from build123d import *

# Parameters (mm, degrees)
SKETCH_1_W          = 120
SKETCH_1_H          = 45
SKETCH_1_R          = 2.6
EXTRUDE_1_DEPTH     = 20
FILLET_1_R          = 10
CUT_EXTRUDE_1_DEPTH = 10


with BuildPart() as part:
    # 草图1 → 凸台-拉伸1 (new body)
    with BuildSketch(Plane.XY):
        Rectangle(SKETCH_1_W, SKETCH_1_H)
        with Locations((-50.8, 12.7)):
            Circle(SKETCH_1_R, mode=Mode.SUBTRACT)
        with Locations((-50.8, 0)):
            Circle(SKETCH_1_R, mode=Mode.SUBTRACT)
        with Locations((-50.8, -12.7)):
            Circle(SKETCH_1_R, mode=Mode.SUBTRACT)
        with Locations((-38.1, 12.7)):
            Circle(SKETCH_1_R, mode=Mode.SUBTRACT)
        with Locations((-38.1, 0)):
            Circle(SKETCH_1_R, mode=Mode.SUBTRACT)
        with Locations((-38.1, -12.7)):
            Circle(SKETCH_1_R, mode=Mode.SUBTRACT)
        with Locations((-25.4, 12.7)):
            Circle(SKETCH_1_R, mode=Mode.SUBTRACT)
        with Locations((-25.4, 0)):
            Circle(SKETCH_1_R, mode=Mode.SUBTRACT)
        with Locations((-25.4, -12.7)):
            Circle(SKETCH_1_R, mode=Mode.SUBTRACT)
        with Locations((-12.7, 12.7)):
            Circle(SKETCH_1_R, mode=Mode.SUBTRACT)
        with Locations((-12.7, 0)):
            Circle(SKETCH_1_R, mode=Mode.SUBTRACT)
        with Locations((-12.7, -12.7)):
            Circle(SKETCH_1_R, mode=Mode.SUBTRACT)
        with Locations((0, 12.7)):
            Circle(SKETCH_1_R, mode=Mode.SUBTRACT)
        Circle(SKETCH_1_R, mode=Mode.SUBTRACT)
        with Locations((0, -12.7)):
            Circle(SKETCH_1_R, mode=Mode.SUBTRACT)
        with Locations((12.7, 12.7)):
            Circle(SKETCH_1_R, mode=Mode.SUBTRACT)
        with Locations((12.7, 0)):
            Circle(SKETCH_1_R, mode=Mode.SUBTRACT)
        with Locations((12.7, -12.7)):
            Circle(SKETCH_1_R, mode=Mode.SUBTRACT)
        with Locations((25.4, 12.7)):
            Circle(SKETCH_1_R, mode=Mode.SUBTRACT)
        with Locations((25.4, 0)):
            Circle(SKETCH_1_R, mode=Mode.SUBTRACT)
        with Locations((25.4, -12.7)):
            Circle(SKETCH_1_R, mode=Mode.SUBTRACT)
        with Locations((38.1, 12.7)):
            Circle(SKETCH_1_R, mode=Mode.SUBTRACT)
        with Locations((38.1, 0)):
            Circle(SKETCH_1_R, mode=Mode.SUBTRACT)
        with Locations((38.1, -12.7)):
            Circle(SKETCH_1_R, mode=Mode.SUBTRACT)
        with Locations((50.8, 12.7)):
            Circle(SKETCH_1_R, mode=Mode.SUBTRACT)
        with Locations((50.8, 0)):
            Circle(SKETCH_1_R, mode=Mode.SUBTRACT)
        with Locations((50.8, -12.7)):
            Circle(SKETCH_1_R, mode=Mode.SUBTRACT)
    extrude(amount=EXTRUDE_1_DEPTH)

    # 圆角1
    fillet_1_edges = [part.edges().sort_by_distance(p)[0] for p in [
        (60, -22.5, 10),
        (-60, -22.5, 10),
        (-60, 22.5, 10),
        (60, 22.5, 10),
    ]]
    fillet(fillet_1_edges, radius=FILLET_1_R)

    # 草图2 → 切除-拉伸1 (cut)
    with BuildSketch(Plane.XY.offset(20)):
        with BuildLine():
            Line((-60, 5.2), (65.881182767, 5.2))
            ThreePointArc((65.881182767, 5.2), (71.081182767, 0), (65.881182767, -5.2))
            Line((65.881182767, -5.2), (-60, -5.2))
            ThreePointArc((-60, -5.2), (-65.2, 0), (-60, 5.2))
        make_face()
    extrude(amount=-CUT_EXTRUDE_1_DEPTH, mode=Mode.SUBTRACT)


solid = part.part
The model under review builds one solid part; all positions refer to its coordinate system, in mm. A direction names the side the tool comes from. Coordinates: 2 decimals unless noted, no trailing zeros. Write each loop counter-clockwise with the first axis right and the second up, starting at its lowest first coordinate (ties: lowest second). Pieces come first, ordered by that corner, then holes. Notation, with made-up numbers: M 44,21.25 L 73,21.25 A15 ccw 73,40.25 Z; hole C 55.25,62.25 d10. An arc over 180 degrees is marked long. Put each result on its own line as item: value.
1) Add section C-C on x = -31. Give the boundary of the cut face in (y, z), then the cut area to 3 significant figures.
Computed:
outline: M -22.5,0 L 22.5,0 L 22.5,20 L 5.2,20 L 5.2,10 L -5.2,10 L -5.2,20 L -22.5,20 Z
area: 796 mm2
2) Add section B-B on x = -12.7. Give the boundary of the cut face in (y, z).
Computed:
outline: M -22.5,0 L -15.3,0 L -15.3,20 L -22.5,20 Z; M -10.1,0 L -2.6,0 L -2.6,10 L -5.2,10 L -5.2,20 L -10.1,20 Z; M 2.6,0 L 10.1,0 L 10.1,20 L 5.2,20 L 5.2,10 L 2.6,10 Z; M 15.3,0 L 22.5,0 L 22.5,20 L 15.3,20 Z
3) Draft analysis for pull direction Y (two halves, no side actions). For faces 1 (the cylindrical face through (-35.62, -11.92, 9.86)), 2 (the flat face through (-1, -22.5, 10)), 3 (the cylindrical face through (-48.32, 0.78, 4.93)), 4 (the flat face through (-1, 22.5, 10)), state which applies: released by +Y, released by -Y, zero draft, split by the parting line, or undercut.
Computed:
face 1: undercut
face 2: released by -Y
face 3: undercut
face 4: released by +Y
4) Wall thickness on probe 1 along Y at (x, z) = (0, 14); probe 2 along Y at (x, z) = (-38.1, 9.25); probe 3 along Y at (x, z) = (-6.5, 16.25): over which ranges is each line inside the solid? List them lowest first. Write a range as [from, to].
Computed:
probe 1: y = [-22.5, -15.3], [-10.1, -5.2], [5.2, 10.1], [15.3, 22.5]
probe 2: y = [-22.5, -15.3], [-10.1, -2.6], [2.6, 10.1], [15.3, 22.5]
probe 3: y = [-22.5, -5.2], [5.2, 22.5]
5) For faces 5 (the cylindrical face through (-23, 1, 5)), 6 (the flat face through (14.2, 2.4, 10)), list the 3-axis set-ups (+Z, -Z, +X, -X, +Y, -Y) from which the entire face can be reached by the end or side of a thin tool; tool diameter is ignored.
Computed:
face 5: +Z, -Z
face 6: +Z, +X, -X
6) Clearance check with a flat-ended pin moving along its axis: pin 1 Ø4 at (y, z) = (15.5, 13) entering from -X. State where the tip first meets the part, or that it passes through.
Computed:
pin 1: stops at x = -59.95
7) Add section A-A on z = 15.5. State how many separate pieces and enclosed holes the cut face has, then the cut area to 3 significant figures.
Computed:
separate pieces: 2
enclosed holes: 18
area: 3,680 mm2
